Geometry check sheet. Reference: drawing and pictorial views, mm from the part's lowest x, y, z. A direction names the side the tool comes from. Give positions to 0.01 mm unless a question says otherwise; leave off trailing zeros. Write each loop counter-clockwise with the first axis right and the second up, starting at its lowest first coordinate (ties: lowest second). Pieces come first, ordered by that corner, then holes. Notation, with made-up numbers: (-37, 72) -> (-27, 72) arc R27 cw to (-27, 89) -> close; hole circle Ø6 at (47, -5). An arc over 180 degrees is marked (long way). Write each question's results on one line, items separated by ' | '. Start each with the question number.
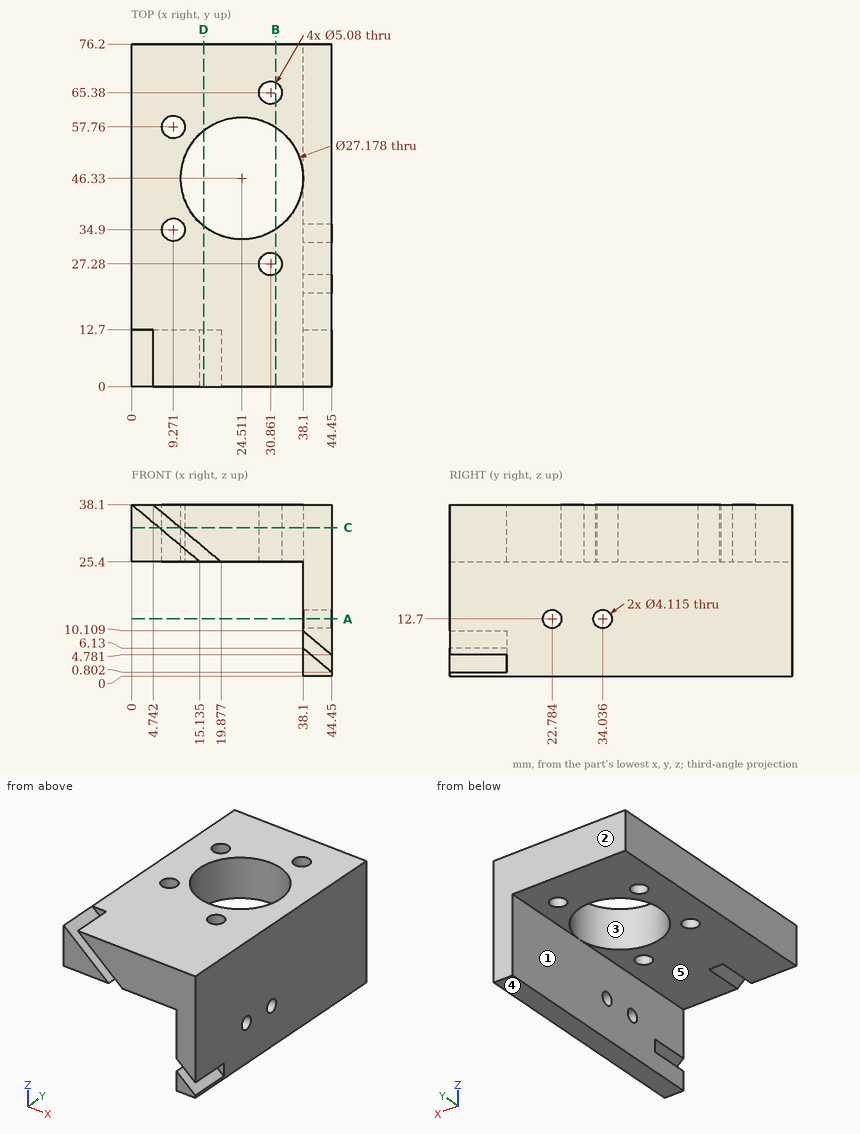
Item 1: Section check D-D on x = 16. Record the boundary of the cut face in (y, z).
Item 2: Thickness scan on probe 1 along Y at (x, z) = (39.75, 12.7); probe 2 along Z at (x, y) = (31, 23); probe 3 along X at (y, z) = (54.5, 22.5). Record the ranges inside material, lowest first. Write a range as from..to.
Item 3: Section check A-A on z = 12.7. Record the boundary of the cut face in (x, y).
Item 4: Section check B-B on x = 32. Record the boundary of the cut face in (y, z).
Item 5: Section check C-C on z = 33. Record the boundary of the cut face in (x, y), then the cut area to 3 significant figures.
Item 6: Mould release check, pull along X, two halves, no side actions. Record for the marked faces 1, 2 and 3: pulls with the +X half, pulls with the -X half, needs draft (parallel to the pull), parting line crosses it, or undercut.
Item 7: Set-up check for the marked faces 4 and 5: record each of +Z, -Z, +X, -X, +Y, -Y from which the full face is reachable in a straight line by a thin tool's end or side.
Item 8: Depth check by flat-ended pin: pin 1 Ø19 at (x, y) = (22, 43) entering from -Z; pin 2 Ø7.5 at (y, z) = (46.5, 12.5) entering from -X. Enter the tip coordinate at first touch or a pass-through.
Check sheet entries:
1) outline: (0, 28.65) -> (12.7, 28.65) -> (12.7, 25.4) -> (35.74, 25.4) -> (35.74, 38.1) -> (0, 38.1) -> close; (56.92, 25.4) -> (76.2, 25.4) -> (76.2, 38.1) -> (56.92, 38.1) -> close
2) probe 1: y = 0..20.73, 24.84..31.98, 36.09..76.2 | probe 2: z = 25.4..38.1 | probe 3: x = 38.1..44.45
3) outline: (38.1, 0) -> (44.45, 0) -> (44.45, 20.73) -> (38.1, 20.73) -> close; (38.1, 24.84) -> (44.45, 24.84) -> (44.45, 31.98) -> (38.1, 31.98) -> close; (38.1, 36.09) -> (44.45, 36.09) -> (44.45, 76.2) -> (38.1, 76.2) -> close
4) outline: (0, 25.4) -> (25.01, 25.4) -> (25.01, 38.1) -> (0, 38.1) -> close; (29.55, 25.4) -> (34.99, 25.4) -> (34.99, 38.1) -> (29.55, 38.1) -> close; (57.67, 25.4) -> (63.11, 25.4) -> (63.11, 38.1) -> (57.67, 38.1) -> close; (67.65, 25.4) -> (76.2, 25.4) -> (76.2, 38.1) -> (67.65, 38.1) -> close
5) outline: (0, 0) -> (6.08, 0) -> (6.08, 12.7) -> (10.82, 12.7) -> (10.82, 0) -> (44.45, 0) -> (44.45, 76.2) -> (0, 76.2) -> close; hole circle Ø5.08 at (9.27, 34.9); hole circle Ø5.08 at (9.27, 57.76); hole circle Ø27.18 at (24.51, 46.33); hole circle Ø5.08 at (30.86, 27.28); hole circle Ø5.08 at (30.86, 65.38) | area: 2,670 mm^2
6) face 1: pulls with the -X half | face 2: needs draft | face 3: undercut
7) face 4: -Z, +X, -X, +Y, -Y | face 5: -Z, -X, +Y, -Y
8) pin 1: stops at z = 25.4 | pin 2: stops at x = 38.1
